For this review, take the finished solid that the model builds, in its own axes (mm). A direction names the side the tool comes from. Round coordinates to 2 decimals unless told otherwise and drop trailing zeros. Write each loop counter-clockwise with the first axis right and the second up, starting at its lowest first coordinate (ties: lowest second). Pieces come first, ordered by that corner, then holes.
from build123d import *

# Parameters (mm, degrees)
BOSS_EXTRUDE1_DEPTH = 127
FILLET1_R           = 31.75


with BuildPart() as part:
    # Sketch1 → Boss-Extrude1 (new body)
    with BuildSketch(Plane(origin=(0, 0, 0), x_dir=(1, 0, 0), z_dir=(0, 1, 0))):
        Polygon((63.5, 63.5), (927.1, 63.5), (927.1, 336.55), (990.6, 336.55), (990.6, 63.5), (990.6, 0), (0, 0), (0, 63.5), (0, 234.95), (63.5, 234.95), align=None)
    extrude(amount=BOSS_EXTRUDE1_DEPTH)

    # Fillet1
    fillet1_edges = [part.edges().sort_by_distance(p)[0] for p in [
        (495.3, 127, 0),
        (990.6, 0, -168.275),
        (495.3, 0, 0),
        (0, 0, -117.475),
        (990.6, 127, -168.275),
        (990.6, 63.5, 0),
        (0, 63.5, 0),
        (0, 127, -117.475),
    ]]
    fillet(fillet1_edges, radius=FILLET1_R)


solid = part.part
(1) We need section D-D, the plane z = -256.5. Give the boundary of the cut face in (x, y).
Geometry check:
outline: (927.1, 0) - (958.85, 0) arc R31.75 ccw to (990.6, 31.75) - (990.6, 95.25) arc R31.75 ccw to (958.85, 127) - (927.1, 127) - close
(2) We need section C-C, the plane x = 441. Give the boundary of the cut face in (y, z).
Geometry check:
outline: (0, -63.5) - (127, -63.5) - (127, -31.75) arc R31.75 ccw to (95.25, 0) - (31.75, 0) arc R31.75 ccw to (0, -31.75) - close
(3) We need section B-B, the plane y = 51.5. Give the boundary of the cut face in (x, z).
Geometry check:
outline: (0, -234.95) - (63.5, -234.95) - (63.5, -63.5) - (927.1, -63.5) - (927.1, -336.55) - (990.6, -336.55) - (990.6, -31.75) arc R31.75 ccw to (958.85, 0) - (31.75, 0) arc R31.75 ccw to (0, -31.75) - close
(4) For line 1 along X through (y, z) = (34, -158); line 2 along X through (y, z) = (29.5, -167); line 3 along Z through (x, y) = (584, 51), list the stretches that pass through material, from the lowest coordinate up.
Geometry check:
line 1: x = 0 to 63.5, 927.1 to 990.6
line 2: x = 0.08 to 63.5, 927.1 to 990.52
line 3: z = -63.5 to 0
(5) We need section A-A, the plane z = -98. Give the boundary of the cut face in (x, y).
Geometry check:
outline: (0, 31.75) arc R31.75 ccw to (31.75, 0) - (63.5, 0) - (63.5, 127) - (31.75, 127) arc R31.75 ccw to (0, 95.25) - close; (927.1, 0) - (958.85, 0) arc R31.75 ccw to (990.6, 31.75) - (990.6, 95.25) arc R31.75 ccw to (958.85, 127) - (927.1, 127) - close
(6) For pin 1 Ø10 at (x, y) = (273, 51) entering from -Z; pin 2 Ø10 at (y, z) = (21, -151.5) entering from -X (3 decimals), all flat-tipped, find the tip position at first contact; note any pin that passes through.
Geometry check:
pin 1: stops at z = -63.5
pin 2: stops at x = 0.525
(7) Mouldability with a two-part tool opening along X and no side actions: class faces 3 (the face through (31, 63, -234.95)), 4 (the face through (489, 63, -63.5)), 5 (the face through (9.1, 9.5, -131.9)) as pulls with the +X half, pulls with the -X half, needs draft (parallel to the pull), parting line crosses it, or undercut.
Geometry check:
face 3: needs draft
face 4: undercut
face 5: pulls with the -X half
(8) For faces 1 (the face through (9.5, 63.9, -9.1)), 2 (the face through (63.5, 63, -150)), list the 3-axis set-ups (+Z, -Z, +X, -X, +Y, -Y) from which the entire face can be reached by the end or side of a thin tool; tool diameter is ignored.
Geometry check:
face 1: +Z, -X, +Y, -Y
face 2: -Z, +Y, -Y
